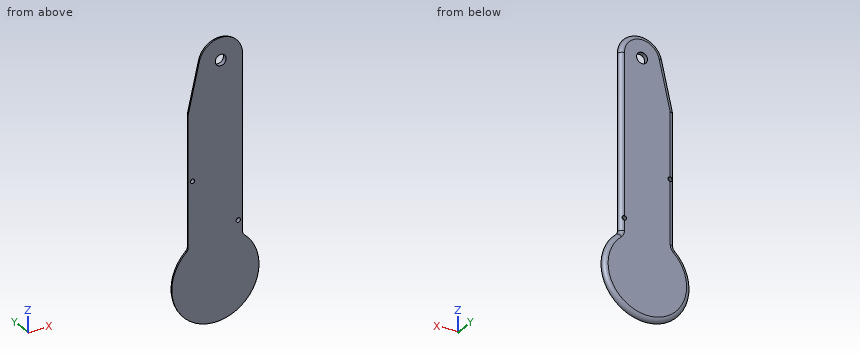
```python
from build123d import *

# Parameters (mm, degrees)
SKETCH1_R           = 3.175
SKETCH1_R_2         = 1.27
BOSS_EXTRUDE1_DEPTH = 2.54
FILLET1_R           = 2.54
FILLET2_R           = 2.54


with BuildPart() as part:
    # Sketch1 → Boss-Extrude1 (new body)
    with BuildSketch(Plane(origin=(0, 0, 0), x_dir=(1, 0, 0), z_dir=(0, 1, 0))):
        with BuildLine():
            Line((-15.875, -19.827868645), (-15.875, -96.027868645))
            Line((-15.875, -96.027868645), (-9.362396438, -124.297332186))
            ThreePointArc((-9.362396438, -124.297332186), (4.537150087, -134.127868645), (15.875, -121.427868645))
            Line((15.875, -121.427868645), (15.875, -96.027868645))
            Line((15.875, -96.027868645), (15.875, -19.827868645))
            ThreePointArc((15.875, -19.827868645), (0, 25.4), (-15.875, -19.827868645))
        make_face()
        with Locations(Location((3.093174395, -121.427868645, 0), (0, 0, 270))):
            Circle(SKETCH1_R, mode=Mode.SUBTRACT)
        with Locations(Location((-13.335, -57.927868645, 0), (0, 0, 270))):
            Circle(SKETCH1_R_2, mode=Mode.SUBTRACT)
        with Locations(Location((13.335, -28.25059986, 0), (0, 0, 270))):
            Circle(SKETCH1_R_2, mode=Mode.SUBTRACT)
    extrude(amount=BOSS_EXTRUDE1_DEPTH)

    # Fillet1
    fillet1_edges = [part.edges().sort_by_distance(p)[0] for p in [
        (15.875, 1.27, 19.827868645),
        (-15.875, 1.27, 96.027868645),
        (-15.875, 1.27, 19.827868645),
    ]]
    fillet(fillet1_edges, radius=FILLET1_R)

    # Fillet2
    # the kernel refuses this fillet: 2.54 mm, written as the material it takes off along each edge
    with BuildSketch(Plane(origin=(-18.415, 2.54, 21.012647977), x_dir=(1, 0, 0), z_dir=(0, 0, 1))) as fillet2_piece_1:
        with BuildLine():
            CenterArc((2.54 + FILLET2_R, -FILLET2_R), FILLET2_R, 90, 90)
            Line((2.54 + FILLET2_R, 0), (2.54, 0))
            Line((2.54, 0), (2.54, -FILLET2_R))
        make_face()
    revolve(axis=Axis((-18.415, 2.54, 21.012647977), (0, 1, 0)), revolution_arc=48.769422845, mode=Mode.SUBTRACT)
    with BuildSketch(Plane(origin=(0, 2.54, 0), x_dir=(0.6590909090909091, 0, 0.7520632776261045), z_dir=(-0.7520632776261045, 0, 0.6590909090909091))) as fillet2_piece_2:
        with BuildLine():
            CenterArc((25.4 - FILLET2_R, -FILLET2_R), FILLET2_R, 0, 90)
            Line((25.4, -FILLET2_R), (25.4, 0))
            Line((25.4, 0), (25.4 - FILLET2_R, 0))
        make_face()
    revolve(axis=Axis((0, 2.54, 0), (0, 1, 0)), revolution_arc=277.53884569, mode=Mode.SUBTRACT)
    with BuildSketch(Plane(origin=(18.415, 2.54, 21.012647977), x_dir=(-1, 0, 0), z_dir=(0, 0, 1))) as fillet2_piece_3:
        with BuildLine():
            CenterArc((2.54 + FILLET2_R, FILLET2_R), FILLET2_R, 180, 90)
            Line((2.54, FILLET2_R), (2.54, 0))
            Line((2.54, 0), (2.54 + FILLET2_R, 0))
        make_face()
    revolve(axis=Axis((18.415, 2.54, 21.012647977), (0, -1, 0)), revolution_arc=48.769422845, mode=Mode.SUBTRACT)
    with BuildSketch(Plane(origin=(15.875, 2.54, 21.012647977), x_dir=(-1, 0, 0), z_dir=(0, 0, 1))) as fillet2_piece_4:
        with BuildLine():
            CenterArc((FILLET2_R, FILLET2_R), FILLET2_R, 180, 90)
            Line((0, FILLET2_R), (0, 0))
            Line((0, 0), (FILLET2_R, 0))
        make_face()
    extrude(amount=100.415220668, mode=Mode.SUBTRACT)
    with BuildSketch(Plane(origin=(3.093174395, 2.54, 121.427868645), x_dir=(-0.9744751037997539, 0, 0.2244955947774008), z_dir=(-0.2244955947774008, 0, -0.9744751037997539))) as fillet2_piece_5:
        with BuildLine():
            CenterArc((12.781825605 - FILLET2_R, -FILLET2_R), FILLET2_R, 0, 90)
            Line((12.781825605, -FILLET2_R), (12.781825605, 0))
            Line((12.781825605, 0), (12.781825605 - FILLET2_R, 0))
        make_face()
    revolve(axis=Axis((3.093174395, 2.54, 121.427868645), (0, 1, 0)), revolution_arc=167.026780897, mode=Mode.SUBTRACT)
    with BuildSketch(Plane(origin=(-15.810166764, 2.54, 96.309292317), x_dir=(0.9744751037997537, 0, -0.22449559477740183), z_dir=(0.22449559477740183, 0, 0.9744751037997537))) as fillet2_piece_6:
        with BuildLine():
            CenterArc((FILLET2_R, -FILLET2_R), FILLET2_R, 90, 90)
            Line((0, -FILLET2_R), (0, 0))
            Line((0, 0), (FILLET2_R, 0))
        make_face()
    extrude(amount=28.721144091, mode=Mode.SUBTRACT)
    with BuildSketch(Plane(origin=(-13.335, 2.54, 95.739073507), x_dir=(-1, 0, 0), z_dir=(0, 0, -1))) as fillet2_piece_7:
        with BuildLine():
            CenterArc((2.54 - FILLET2_R, -FILLET2_R), FILLET2_R, 0, 90)
            Line((2.54 - FILLET2_R, 0), (2.54, 0))
            Line((2.54, 0), (2.54, -FILLET2_R))
        make_face()
    revolve(axis=Axis((-13.335, 2.54, 95.739073507), (0, 1, 0)), revolution_arc=12.973219103, mode=Mode.SUBTRACT)
    with BuildSketch(Plane(origin=(-15.875, 2.54, 21.012647977), x_dir=(0, -1, 0), z_dir=(0, 0, 1))) as fillet2_piece_8:
        with BuildLine():
            CenterArc((FILLET2_R, FILLET2_R), FILLET2_R, 180, 90)
            Line((0, FILLET2_R), (0, 0))
            Line((0, 0), (FILLET2_R, 0))
        make_face()
    extrude(amount=74.72642553, mode=Mode.SUBTRACT)


solid = part.part
```
For this review, take the finished solid that the model builds, in its own axes (mm). Give positions to 0.01 mm unless a question says otherwise; leave off trailing zeros. Order: outer loops, then holes, each group sorted by start corner. A loop starts at its lowest first (then second) coordinate and runs counter-clockwise, first axis right, second up.
1) Insertion check: pin 1 (2 mm diameter, centred on x = -13.34, z = 57.93, fed in from +Y); pin 2 (4 mm diameter, centred on x = 13.5, z = 15.5, fed in from -Y); pin 3 (1.5 mm diameter, centred on y = 2, z = 82.5, fed in from +X). Each pin has a flat end and moves straight along its axis. Give the tip position at first contact, or say it passes through.
2) Wall thickness on line 1 (Z direction, x = -20.5, y = 1.05); line 2 (X direction, y = 2.2, z = 90.5); line 3 (Z direction, x = 4.5, y = 0.9): over which ranges is each line inside the solid? List them lowest first.
3) Take a section at B-B (z = 32.5). Give the boundary of the cut face in (x, y) (3 decimals), then the cut area to 3 significant figures.
4) Take a section at A-A (y = 1.95). State how many separate pieces and enclosed holes the cut face has, then the cut area to 3 significant figures.
Derived:
1. pin 1: passes through
1. pin 2: stops at y = 0
1. pin 3: stops at x = 15.55
2. line 1: z = -14.61 to 14.61
2. line 2: x = -14.6 to 14.6
2. line 3: z = -24.83 to 118.58, 124.27 to 133.97
3. outline: (-15.875, 0) - (15.875, 0) arc R2.54 ccw to (13.335, 2.54) - (-13.335, 2.54) arc R2.54 ccw to start
3. area: 77.9 mm2
4. separate pieces: 1
4. enclosed holes: 3
4. area: 4,940 mm2
